Answer from the drawing. Dimensions are ordinates in mm from the lowest x, y and z of the part. A direction names the side the tool comes from. Give positions to 0.01 mm unless a question says otherwise; leave off trailing zeros. Loops run counter-clockwise (first coordinate to the right, second up) from the corner with the lowest first, then second, coordinate; pieces in that order, holes last. Notation, with made-up numbers: (78, 22.25) - (123, 22.25) arc R18 cw to (123, 50.25) - close; hole circle Ø2 at (23, 87). An arc over 180 degrees is marked (long way). Write each question's results on one line, items separated by ' | '. Start each with the question number.
Q1. The part is cut by section A-A, the plane z = 14. Write down the section's boundary in (x, y).
Q2. For the marked faces 4, 5, 6, 7 and 8, determine the directions among +Z, -Z, +X, -X, +Y, -Y from which every point of the face is accessible in a straight line to the end or side of a thin tool.
Q3. The part is cut by section D-D, the plane z = 33.5. Write down the section's boundary in (x, y).
Q4. The part is cut by section C-C, the plane y = 6.5. Write down the section's boundary in (x, z).
Q5. Given pin 1 (3 mm diameter, centred on y = 3.5, z = 36.5, fed in from -X); pin 2 (5 mm diameter, centred on x = 10.5, y = 2.5, fed in from +Z); pin 3 (3 mm diameter, centred on x = 22.5, y = 5, fed in from +Z), each flat-ended and moving along its own axis, determine where each tip first touches the part or whether it passes through.
Q6. Determine the mould class of the marked faces 1, 2 and 3 for opening direction X: +X half, -X half, draft (parallel to the pull), parting line (faces both ways), or undercut.
Q7. Find the intervals of material crossed by line 1 (X direction, y = 8, z = 12); line 2 (X direction, y = 1.75, z = 34.5); line 3 (Z direction, x = 11, y = 2), in increasing order. Write a range as from..to.
Q8. The part is cut by section B-B, the plane x = 24.5. Write down the section's boundary in (y, z).
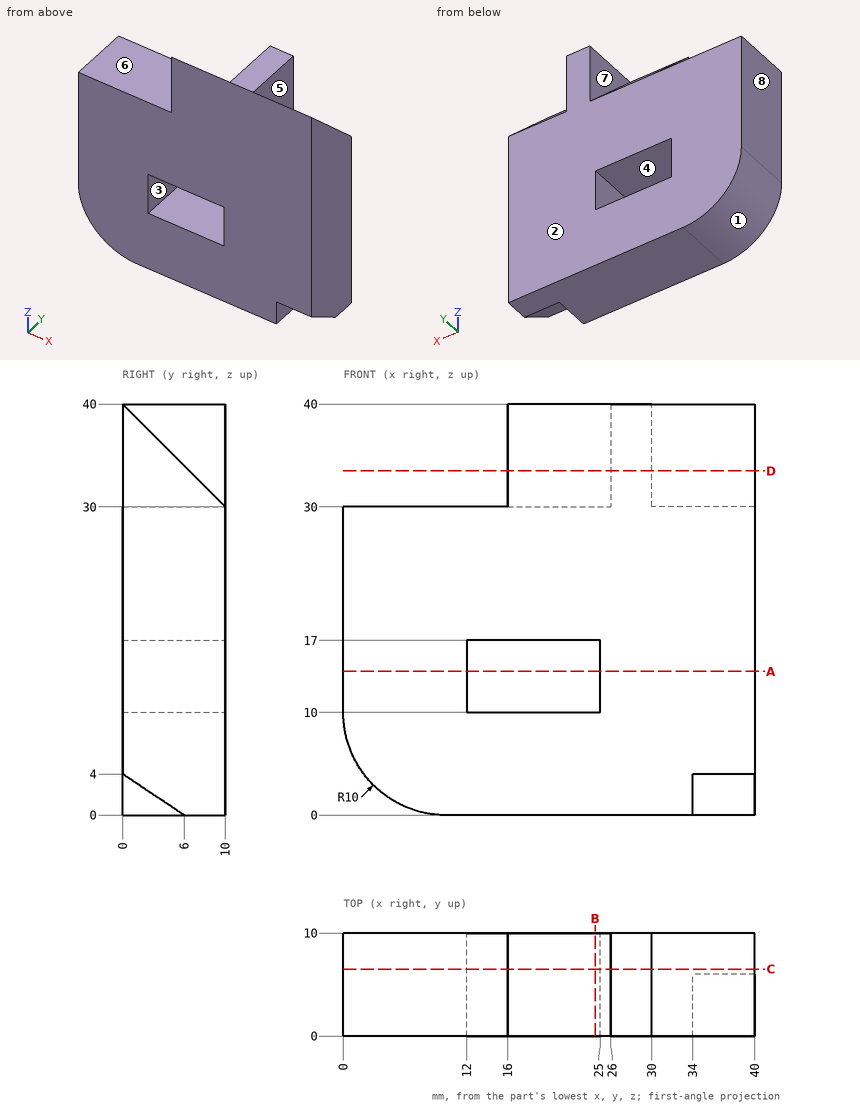
Check sheet entries:
1) outline: (0, 0) - (12, 0) - (12, 10) - (0, 10) - close; (25, 0) - (40, 0) - (40, 10) - (25, 10) - close
2) face 4: +Y, -Y | face 5: +Z, +X, +Y | face 6: +Z, -X, +Y, -Y | face 7: +Z, -X, +Y | face 8: +Z, -Z, -X, +Y, -Y
3) outline: (16, 0) - (40, 0) - (40, 6.5) - (30, 6.5) - (30, 10) - (26, 10) - (26, 6.5) - (16, 6.5) - close
4) outline: (0, 10) arc R10 ccw to (10, 0) - (40, 0) - (40, 33.5) - (30, 33.5) - (30, 40) - (26, 40) - (26, 33.5) - (16, 33.5) - (16, 30) - (0, 30) - close; hole (12, 10) - (25, 10) - (25, 17) - (12, 17) - close
5) pin 1: stops at x = 16 | pin 2: stops at z = 30 | pin 3: stops at z = 36.5
6) face 1: -X half | face 2: draft | face 3: undercut
7) line 1: x = 0..12, 25..40 | line 2: x = 16..40 | line 3: z = 0..30
8) outline: (0, 0) - (10, 0) - (10, 10) - (0, 10) - close; (0, 17) - (10, 17) - (10, 30) - (0, 40) - close
